Geometry check sheet. Reference: the model listing, model coordinates, mm. A direction names the side the tool comes from. Coordinates: 2 decimals unless noted, no trailing zeros. Order: outer loops, then holes, each group sorted by start corner. A loop starts at its lowest first (then second) coordinate and runs counter-clockwise, first axis right, second up. Notation, with made-up numbers: (-29.75, 59) - (-5.75, 59) arc R6 ccw to (-5.75, 65) - close; hole circle Ø5 at (-36, 48). An arc over 180 degrees is marked (long way). Return JSON: item names as keys, results as strings. Group by question number.
Item 1: Draft check along Z on faces 3 (the cylindrical face through (67.6, -12.5, 4.3)), 4 (the flat face through (22, 0, 0)), 5 (the cylindrical face through (-28.57, -25.04, 0.63)). Enter one of: pulls with the +Z half, pulls with the -Z half, needs draft (parallel to the pull), parting line crosses it, or undercut.
Item 2: Tool access check on faces 1 (the flat face through (-13, -50.8, 7)), 2 (the flat face through (16, -25, 4.762)). Record the directions out of +Z, -Z, +X, -X, +Y, -Y that give a thin tool (end or side, any length) a straight path to the whole face; none if there is none.
Item 3: Section check C-C on x = 50. Enter the section's corners in (y, z).
Item 4: Section check B-B on z = -8. Enter the section's corners in (x, y).
Item 5: Gauge pin test, flat ends, axial feed: pin 1 (3 mm diameter, centred on x = 15, y = -35, fed in from +Z); pin 2 (2 mm diameter, centred on y = -12, z = 3, fed in from +X); pin 3 (12 mm diameter, centred on x = 31.5, y = -19.5, fed in from +Z). Record the tip position at first contact, or that the pin passes through.
Item 6: Section check D-D on y = -4.5. Give the number of separate pieces and of enclosed holes in the cut face, then the cut area to 3 significant figures.
Item 7: Scan lines: probe 1 along X at (y, z) = (-20, 1); probe 2 along X at (y, z) = (-25, 12.5); probe 3 along Z at (x, y) = (16.5, -43). Record each from-to range of solid material in increasing order.
from build123d import *

# Parameters (mm, degrees)
F0_R     = 14.2875
F1_DEPTH = 25.4
F2_DEPTH = 50.8


with BuildPart() as f1:
    # F0 (on Front) → F1 (new body)
    with BuildSketch(Plane.XZ):
        with BuildLine():
            Line((9.5121844836, 26.9452959039), (0, 28.575))
            ThreePointArc((0, 28.575), (-28.575, 0), (0, -28.575))
            Line((0, -28.575), (9.5121844836, -26.9452959039))
            ThreePointArc((9.5121844836, -26.9452959039), (23.3274655355, -16.5033322905), (28.575, 0))
            ThreePointArc((28.575, 0), (23.3274655355, 16.5033322905), (9.5121844836, 26.9452959039))
        make_face()
        with BuildLine():
            ThreePointArc((-13.4703841816, 4.7625), (0, 14.2875), (13.4703841816, 4.7625))
            Line((13.4703841816, 4.7625), (19.05, 4.7625))
            Line((19.05, 4.7625), (19.05, -4.7625))
            Line((19.05, -4.7625), (13.4703841816, -4.7625))
            ThreePointArc((13.4703841816, -4.7625), (0, -14.2875), (-13.4703841816, -4.7625))
            Line((-13.4703841816, -4.7625), (-19.05, -4.7625))
            Line((-19.05, -4.7625), (-19.05, 4.7625))
            Line((-19.05, 4.7625), (-13.4703841816, 4.7625))
        make_face(mode=Mode.SUBTRACT)
        with BuildLine():
            Line((57.1919272622, 18.7764181619), (9.5121844836, 26.9452959039))
            ThreePointArc((9.5121844836, 26.9452959039), (23.3274655355, 16.5033322905), (28.575, 0))
            ThreePointArc((28.575, 0), (23.3274655355, -16.5033322905), (9.5121844836, -26.9452959039))
            Line((9.5121844836, -26.9452959039), (57.1919272622, -18.7764181619))
            ThreePointArc((57.1919272622, -18.7764181619), (34.925, 0), (57.1919272622, 18.7764181619))
        make_face()
        with BuildLine():
            ThreePointArc((73.025, 0), (68.5383952831, 12.2804730295), (57.1919272622, 18.7764181619))
            ThreePointArc((57.1919272622, 18.7764181619), (34.925, 0), (57.1919272622, -18.7764181619))
            ThreePointArc((57.1919272622, -18.7764181619), (68.5383952831, -12.2804730295), (73.025, 0))
        make_face()
        with Locations((53.975, 0)):
            Circle(F0_R, mode=Mode.SUBTRACT)
        with BuildLine():
            ThreePointArc((-13.4703841816, -4.7625), (-14.2875, 0), (-13.4703841816, 4.7625))
            Line((-13.4703841816, 4.7625), (-19.05, 4.7625))
            Line((-19.05, 4.7625), (-19.05, -4.7625))
            Line((-19.05, -4.7625), (-13.4703841816, -4.7625))
        make_face()
    extrude(amount=F1_DEPTH)

    # F0 (on Front) → F2 (join)
    with BuildSketch(Plane.XZ):
        with BuildLine():
            Line((9.5121844836, 26.9452959039), (0, 28.575))
            ThreePointArc((0, 28.575), (-28.575, 0), (0, -28.575))
            Line((0, -28.575), (9.5121844836, -26.9452959039))
            ThreePointArc((9.5121844836, -26.9452959039), (23.3274655355, -16.5033322905), (28.575, 0))
            ThreePointArc((28.575, 0), (23.3274655355, 16.5033322905), (9.5121844836, 26.9452959039))
        make_face()
        with BuildLine():
            ThreePointArc((-13.4703841816, 4.7625), (0, 14.2875), (13.4703841816, 4.7625))
            Line((13.4703841816, 4.7625), (19.05, 4.7625))
            Line((19.05, 4.7625), (19.05, -4.7625))
            Line((19.05, -4.7625), (13.4703841816, -4.7625))
            ThreePointArc((13.4703841816, -4.7625), (0, -14.2875), (-13.4703841816, -4.7625))
            Line((-13.4703841816, -4.7625), (-19.05, -4.7625))
            Line((-19.05, -4.7625), (-19.05, 4.7625))
            Line((-19.05, 4.7625), (-13.4703841816, 4.7625))
        make_face(mode=Mode.SUBTRACT)
        with BuildLine():
            ThreePointArc((-13.4703841816, -4.7625), (-14.2875, 0), (-13.4703841816, 4.7625))
            Line((-13.4703841816, 4.7625), (-19.05, 4.7625))
            Line((-19.05, 4.7625), (-19.05, -4.7625))
            Line((-19.05, -4.7625), (-13.4703841816, -4.7625))
        make_face()
    extrude(amount=F2_DEPTH)


solid = f1.part
Computed:
{
 "1": {"face 3": "undercut", "face 4": "needs draft", "face 5": "parting line crosses it"},
 "2": {"face 1": "+Z, -Z, +X, -X, -Y", "face 2": "+Y, -Y"},
 "3": {"outline": "(-25.4, -20.01) - (0, -20.01) - (0, -13.72) - (-25.4, -13.72) - close; (-25.4, 13.72) - (0, 13.72) - (0, 20.01) - (-25.4, 20.01) - close"},
 "4": {"outline": "(-27.43, -50.8) - (-11.84, -50.8) - (-11.84, 0) - (-27.43, 0) - close; (11.84, -50.8) - (27.43, -50.8) - (27.43, -25.4) - (42.14, -25.4) - (42.14, 0) - (11.84, 0) - close; (65.81, -25.4) - (71.26, -25.4) - (71.26, 0) - (65.81, 0) - close"},
 "5": {"pin 1": "stops at z = 25.18", "pin 2": "stops at x = 72.92", "pin 3": "stops at z = 24.21"},
 "6": {"separate pieces": "1", "enclosed holes": "2", "area": "3,110 mm²"},
 "7": {"probe 1": "x = -28.56 to -14.25, 19.05 to 39.72, 68.23 to 73", "probe 2": "x = -25.7 to -6.92, 6.92 to 47.06, 60.89 to 68.35", "probe 3": "z = -23.33 to -4.76, 4.76 to 23.33"}
}
